Check sheet for the modelled part. Datum: model origin and axes. Units: mm. Face numbers are marked on the shaded views. A direction names the side the tool comes from. Round coordinates to 2 decimals unless told otherwise and drop trailing zeros. Write each loop counter-clockwise with the first axis right and the second up, starting at its lowest first coordinate (ties: lowest second). Pieces come first, ordered by that corner, then holes. Notation, with made-up numbers: (50, 48) -> (108, 48) arc R21 ccw to (108, 54) -> close; hole circle Ø7 at (32.25, 75.5). An arc over 180 degrees is marked (long way). One line per item, written item: value.
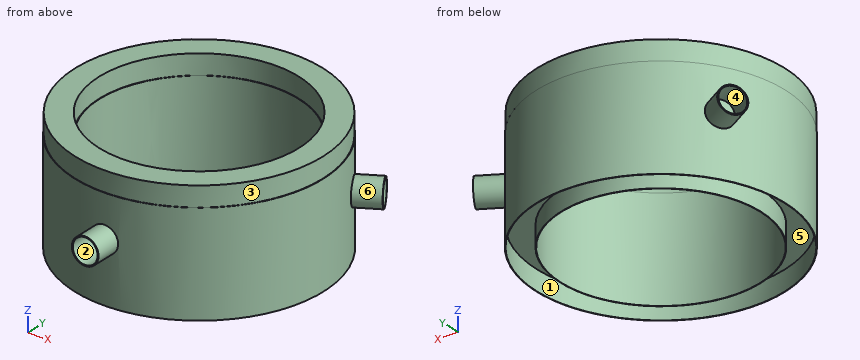
from build123d import *

# Parameters (mm, degrees)
F2_R     = 25
F3_DEPTH = 661
F5_R     = 27
F5_R_2   = 25
F6_DEPTH = 50
F7_COUNT = 3


with BuildPart() as f1:
    # F0 (on Front) → F1 (revolve)
    with BuildSketch(Plane.XZ):
        Polygon((-201, -489.7526234735), (-200, -489.7526234735), (-200, -284.7526234735), (-201, -284.7526234735), (-201, -244.7526234735), (-249, -244.7526234735), (-249, -284.7526234735), (-250, -284.7526234735), (-250, -489.7526234735), (-249, -489.7526234735), (-249, -449.7526234735), (-201, -449.7526234735), align=None)
    revolve(axis=Axis((0, 0, -77.0492781825), (0, 0, -1)))

    # F2 (on Front) → F3 (cut)
    with BuildSketch(Plane.XZ):
        with Locations((0, -369.7526234735)):
            Circle(F2_R)
    extrude(amount=F3_DEPTH, mode=Mode.SUBTRACT)

    # F5 (on offset) → F6 (join, symmetric)
    with BuildSketch(Plane.XZ.offset(250)):
        with Locations((0, -369.7526234735)):
            Circle(F5_R)
        with Locations((0, -369.7526234735)):
            Circle(F5_R_2, mode=Mode.SUBTRACT)
    extrude(amount=F6_DEPTH, both=True)

    # F7: F1 ×3 about axis
    f7_axis = Axis((0, 0, -369.7526234735), (0, 0, -1))


with BuildPart() as f1_1:
    add(f1.part)
    for i in range(1, F7_COUNT):
        add(f1.part.rotate(f7_axis, i * 360 / F7_COUNT))


solid = f1_1.part
Item 1: Release check for a two-part mould opening along Z. For the marked faces 4, 5 and 6 record: pulls with the +Z half, pulls with the -Z half, needs draft (parallel to the pull), parting line crosses it, or undercut.
Result set:
face 4: undercut
face 5: pulls with the -Z half
face 6: parting line crosses it
Item 2: Sectioned sample at A-A (y = 0). Enter the section's corners in (x, z), then the cut area to 3 significant figures.
Result set:
outline: (-250, -489.75) -> (-249, -489.75) -> (-249, -449.75) -> (-201, -449.75) -> (-201, -489.75) -> (-200, -489.75) -> (-200, -284.75) -> (-201, -284.75) -> (-201, -244.75) -> (-249, -244.75) -> (-249, -284.75) -> (-250, -284.75) -> close; (200, -489.75) -> (201, -489.75) -> (201, -449.75) -> (249, -449.75) -> (249, -489.75) -> (250, -489.75) -> (250, -284.75) -> (249, -284.75) -> (249, -244.75) -> (201, -244.75) -> (201, -284.75) -> (200, -284.75) -> close
area: 20,500 mm^2
Item 3: Material ranges on line 1 along Y through (x, z) = (0, -459); line 2 along X through (y, z) = (0, -443.5); line 3 along Z through (x, y) = (0, -267), recorded low to high.
Result set:
line 1: -250 to -249, -201 to -200, 200 to 201, 249 to 250
line 2: -250 to -200, 200 to 250
line 3: -396.75 to -394.75, -344.75 to -342.75
Item 4: Sectioned sample at B-B (x = 65.5). Enter the section's corners in (y, z).
Result set:
outline: (-241.27, -489.75) -> (-240.23, -489.75) -> (-240.23, -449.75) -> (-190.03, -449.75) -> (-190.03, -489.75) -> (-188.97, -489.75) -> (-188.97, -284.75) -> (-190.03, -284.75) -> (-190.03, -244.75) -> (-240.23, -244.75) -> (-240.23, -284.75) -> (-241.27, -284.75) -> close; (188.97, -489.75) -> (190.03, -489.75) -> (190.03, -449.75) -> (240.23, -449.75) -> (240.23, -489.75) -> (241.27, -489.75) -> (241.27, -284.75) -> (240.23, -284.75) -> (240.23, -244.75) -> (190.03, -244.75) -> (190.03, -284.75) -> (188.97, -284.75) -> close
Item 5: Tool access check on the marked faces 1, 2 and 3. Record the directions out of +Z, -Z, +X, -X, +Y, -Y that give a thin tool (end or side, any length) a straight path to the whole face; none if there is none.
Result set:
face 1: -Z
face 2: -Y
face 3: +Z
Item 6: Sectioned sample at C-C (z = -303.5). Enter the section's corners in (x, y), then the cut area to 3 significant figures.
Result set:
outline: circle Ø500 at (0, 0); hole circle Ø400 at (0, 0)
area: 70,700 mm^2
Item 7: Depth check by flat-ended pin: pin 1 (12 mm diameter, centred on x = -191.5, z = -311, fed in from +Y); pin 2 (1.5 mm diameter, centred on y = 110.5, z = -409.5, fed in from +X); pin 3 (12 mm diameter, centred on y = -173.5, z = -461, fed in from +X). Enter the tip coordinate at first touch or a pass-through.
Result set:
pin 1: y = 167.6
pin 2: x = 224.62
pin 3: x = 185.59
